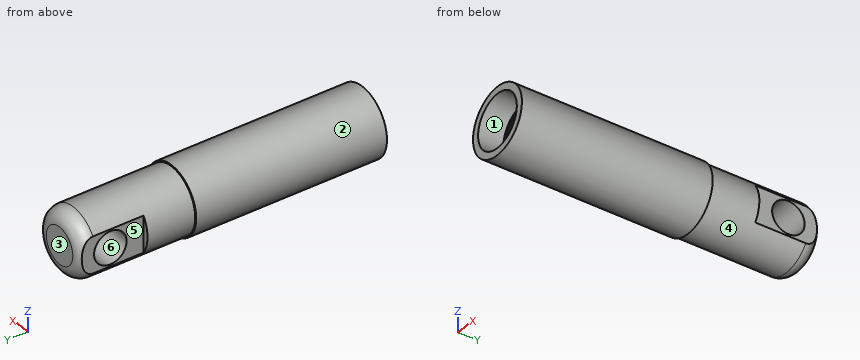
```python
from build123d import *

# Parameters (mm, degrees)
SKETCH1_R           = 11.5
BOSS_EXTRUDE1_DEPTH = 108
FILLET1_R           = 5
SKETCH2_R           = 9.5
CUT_EXTRUDE1_DEPTH  = 80
CUT_EXTRUDE5_START  = -23
CUT_EXTRUDE5_DEPTH  = 23
SKETCH6_R           = 10.5
CUT_EXTRUDE7_DEPTH  = 1
SKETCH8_R           = 12
SKETCH8_R_2         = 11.5
BOSS_EXTRUDE2_DEPTH = 68
SKETCH9_R           = 5.8
CUT_EXTRUDE8_DEPTH  = 111.771160604


with BuildPart() as part:
    # Sketch1 → Boss-Extrude1 (new body)
    with BuildSketch(Plane(origin=(0, 0, 0), x_dir=(1, 0, 0), z_dir=(0, 1, 0))):
        with Locations(Location((0, 0, 0), (0, 0, 270))):
            Circle(SKETCH1_R)
    extrude(amount=BOSS_EXTRUDE1_DEPTH)

    # Fillet1
    fillet1_edges = [part.edges().sort_by_distance(p)[0] for p in [
        (0, 108, -11.5),
    ]]
    fillet(fillet1_edges, radius=FILLET1_R)

    # Sketch2 → Cut-Extrude1 (cut)
    with BuildSketch(Plane.XZ):
        with Locations(Location((0, 0, 0), (0, 0, 270))):
            Circle(SKETCH2_R)
    extrude(amount=-CUT_EXTRUDE1_DEPTH, mode=Mode.SUBTRACT)

    # Sketch3 → Cut-Extrude5 (cut)
    with BuildSketch(Plane(origin=(0, 108, 0), x_dir=(1, 0, 0), z_dir=(0, 1, 0)).offset(CUT_EXTRUDE5_START)):
        with BuildLine():
            Line((-9.5, 6.480740698), (-9.5, -6.480740698))
            ThreePointArc((-9.5, -6.480740698), (-11.5, 0), (-9.5, 6.480740698))
        make_face()
        with BuildLine():
            Line((9.5, 6.480740698), (9.5, -6.480740698))
            ThreePointArc((9.5, -6.480740698), (11.5, 0), (9.5, 6.480740698))
        make_face()
    extrude(amount=CUT_EXTRUDE5_DEPTH, mode=Mode.SUBTRACT)

    # Sketch6 → Cut-Extrude7 (cut)
    with BuildSketch(Plane.XZ.offset(-10)):
        with Locations(Location((0, 0, 0), (0, 0, 270))):
            Circle(SKETCH6_R)
    extrude(amount=CUT_EXTRUDE7_DEPTH, mode=Mode.SUBTRACT)

    # Sketch8 → Boss-Extrude2 (add)
    with BuildSketch(Plane.XZ):
        with Locations(Location((0, 0, 0), (0, 0, 270))):
            Circle(SKETCH8_R)
        with Locations(Location((0, 0, 0), (0, 0, 270))):
            Circle(SKETCH8_R_2, mode=Mode.SUBTRACT)
    extrude(amount=-BOSS_EXTRUDE2_DEPTH)

    # Sketch9 → Cut-Extrude8 (cut, through all)
    with BuildSketch(Plane.ZY.offset(9.5)):
        with Locations((0, 96.8)):
            Circle(SKETCH9_R)
    extrude(amount=-CUT_EXTRUDE8_DEPTH, mode=Mode.SUBTRACT)


solid = part.part
```
Input: part model. Units: mm. Frame: model coordinates. Face numbers are marked on the shaded views. A direction names the side the tool comes from. Coordinates: 2 decimals unless noted, no trailing zeros. Loops run counter-clockwise (first coordinate to the right, second up) from the corner with the lowest first, then second, coordinate; pieces in that order, holes last.
Q1. Set-up query: the marked faces 4, 5 and 6. Return all of +Z, -Z, +X, -X, +Y, -Y with unobstructed straight access to the full face (end or side cutting, diameter ignored); none if empty.
Results are:
face 4: +Y
face 5: +Z, -Z, -X, +Y
face 6: +X, -X
Q2. Section B-B, the plane x = 0. Return the cut outline in (y, z), and give its area (3 significant figures).
Results are:
outline: (0, -12) - (68, -12) - (68, -11.5) - (103, -11.5) arc R5 ccw to (108, -6.5) - (108, 6.5) arc R5 ccw to (103, 11.5) - (68, 11.5) - (68, 12) - (0, 12) - (0, 9.5) - (9, 9.5) - (9, 10.5) - (10, 10.5) - (10, 9.5) - (80, 9.5) - (80, -9.5) - (10, -9.5) - (10, -10.5) - (9, -10.5) - (9, -9.5) - (0, -9.5) - close; hole circle Ø11.6 at (96.8, 0)
area: 914 mm2
Q3. Line query: line 1 along Y through (x, z) = (3, 0); line 2 along X through (y, z) = (2.5, 0); line 3 along Z through (x, y) = (4.5, 21.5). Output: solid intervals per line, ascending.
Results are:
line 1: y = 80 to 91, 102.6 to 108
line 2: x = -12 to -9.5, 9.5 to 12
line 3: z = -11.12 to -8.37, 8.37 to 11.12
Q4. Mould query, pull axis X, two halves, no side actions, for the marked faces 1, 2 and 3. Classes: +X half, -X half, draft (parallel to the pull), parting line (faces both ways), or undercut.
Results are:
face 1: undercut
face 2: parting line
face 3: draft
Q5. Section A-A, the plane y = 96.8. Return the cut outline in (x, z), and give its area (3 significant figures).
Results are:
outline: (-9.5, -6.48) arc R11.5 ccw to (9.5, -6.48) - (9.5, -5.8) - (-9.5, -5.8) - close; (-9.5, 5.8) - (9.5, 5.8) - (9.5, 6.48) arc R11.5 ccw to (-9.5, 6.48) - close
area: 160 mm2
Q6. Contact query for flat-ended pins moving along their axis: pin 1 (11.5 mm diameter, centred on x = 0, z = 0, fed in from -Y); pin 2 (8 mm diameter, centred on y = 38.5, z = -3.5, fed in from -X); pin 3 (0.6 mm diameter, centred on x = -11, z = -2.5, fed in from +Y); pin 4 (8 mm diameter, centred on x = -8.5, y = 33.5, fed in from +Z). Output: stop coordinate, or through.
Results are:
pin 1: stops at y = 80
pin 2: stops at x = -12
pin 3: stops at y = 85
pin 4: stops at z = 11.12
Q7. Section D-D, the plane y = 25.5. Return the cut outline in (x, z).
Results are:
outline: circle Ø24 at (0, 0); hole circle Ø19 at (0, 0)
